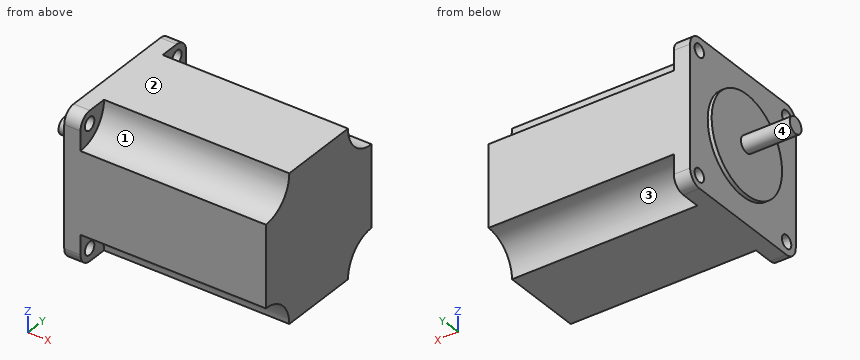
from build123d import *

# Parameters (mm, degrees)
SKETCH1_W           = 57.15
SKETCH1_H           = 57.15
SKETCH1_R           = 2.54
BOSS_EXTRUDE1_DEPTH = 6.35
FILLET1_R           = 5.08
SKETCH5_R           = 19.05
BOSS_EXTRUDE4_DEPTH = 1.524
SKETCH6_R           = 3.175
BOSS_EXTRUDE5_DEPTH = 19.05
BOSS_EXTRUDE6_DEPTH = 72.39


with BuildPart() as part:
    # Sketch1 → Boss-Extrude1 (new body)
    with BuildSketch(Plane(origin=(0, 0, 0), x_dir=(0, 0, -1), z_dir=(1, 0, 0))):
        Rectangle(SKETCH1_W, SKETCH1_H)
        with Locations((23.622, 23.622)):
            Circle(SKETCH1_R, mode=Mode.SUBTRACT)
        with Locations((-23.622, 23.622)):
            Circle(SKETCH1_R, mode=Mode.SUBTRACT)
        with Locations((-23.622, -23.622)):
            Circle(SKETCH1_R, mode=Mode.SUBTRACT)
        with Locations((23.622, -23.622)):
            Circle(SKETCH1_R, mode=Mode.SUBTRACT)
    extrude(amount=BOSS_EXTRUDE1_DEPTH)

    # Fillet1
    fillet1_edges = [part.edges().sort_by_distance(p)[0] for p in [
        (3.175, 28.575, 28.575),
        (3.175, 28.575, -28.575),
        (3.175, -28.575, -28.575),
        (3.175, -28.575, 28.575),
    ]]
    fillet(fillet1_edges, radius=FILLET1_R)

    # Sketch5 → Boss-Extrude4 (add)
    with BuildSketch(Plane.ZY):
        Circle(SKETCH5_R)
    extrude(amount=BOSS_EXTRUDE4_DEPTH)

    # Sketch6 → Boss-Extrude5 (add)
    with BuildSketch(Plane.ZY.offset(1.524)):
        Circle(SKETCH6_R)
    extrude(amount=BOSS_EXTRUDE5_DEPTH)

    # Sketch7 → Boss-Extrude6 (add)
    with BuildSketch(Plane(origin=(6.35, 0, 0), x_dir=(0, 0, -1), z_dir=(1, 0, 0))):
        with BuildLine():
            Line((-15.875, 28.575), (15.875, 28.575))
            ThreePointArc((15.875, 28.575), (19.594743879, 19.594743879), (28.575, 15.875))
            Line((28.575, 15.875), (28.575, -15.875))
            ThreePointArc((28.575, -15.875), (19.594743879, -19.594743879), (15.875, -28.575))
            Line((15.875, -28.575), (-15.875, -28.575))
            ThreePointArc((-15.875, -28.575), (-19.594743879, -19.594743879), (-28.575, -15.875))
            Line((-28.575, -15.875), (-28.575, 15.875))
            ThreePointArc((-28.575, 15.875), (-19.594743879, 19.594743879), (-15.875, 28.575))
        make_face()
    extrude(amount=BOSS_EXTRUDE6_DEPTH)


solid = part.part
Could you check a few things on this model? Use its own coordinates, in mm. Face numbers are marked on the shaded views. A direction names the side the tool comes from. Give positions to 0.01 mm unless a question says otherwise; leave off trailing zeros. Write each loop counter-clockwise with the first axis right and the second up, starting at its lowest first coordinate (ties: lowest second). Pieces come first, ordered by that corner, then holes. Notation, with made-up numbers: (21, 10.5) -> (51, 10.5) arc R6 cw to (51, 15.5) -> close; hole circle Ø11 at (59.25, -33.5). An arc over 180 degrees is marked (long way). Answer as a JSON object with one key per item and string values.
Q1. Will these pins go through, and if not, where does the flat tip stop? pin 1 Ø10 at (y, z) = (9, 2) entering from -X; pin 2 Ø1.5 at (y, z) = (9, 19.5) entering from -X; pin 3 Ø14 at (y, z) = (-23.5, 23.5) entering from +X; pin 4 Ø4 at (x, y) = (53.5, -21.5) entering from +Z.
Taken from the geometry:
{"pin 1": "stops at x = -1.52", "pin 2": "stops at x = 0", "pin 3": "stops at x = 78.74", "pin 4": "stops at z = 19.69"}
Q2. Which directions (+Z, -Z, +X, -X, +Y, -Y) give clear straight access to the entire face, cutting with the end or side of a thin tool? Please do the marked faces 1, 2, 3 and 4.
Taken from the geometry:
{"face 1": "+Z, +X, -Y", "face 2": "+Z, +X, -X, +Y, -Y", "face 3": "-Z, +X, +Y", "face 4": "-X"}
Q3. Suppose I cut it at C-C on z = 8.5. Write out the boundary of the cut face in (x, y) (3 decimals), then the cut area to 3 significant figures.
Taken from the geometry:
{"outline": "(-1.524, -17.049) -> (0, -17.049) -> (0, -28.575) -> (78.74, -28.575) -> (78.74, 28.575) -> (0, 28.575) -> (0, 17.049) -> (-1.524, 17.049) -> close", "area": "4,550 mm²"}
Q4. Suppose I cut it at A-A on y = 0. Write out the boundary of the cut face in (x, z) (3 decimals), then the cut area to 3 significant figures.
Taken from the geometry:
{"outline": "(-20.574, -3.175) -> (-1.524, -3.175) -> (-1.524, -19.05) -> (0, -19.05) -> (0, -28.575) -> (78.74, -28.575) -> (78.74, 28.575) -> (0, 28.575) -> (0, 19.05) -> (-1.524, 19.05) -> (-1.524, 3.175) -> (-20.574, 3.175) -> close", "area": "4,680 mm²"}
Q5. Please list where these lines run through material, in increasing order: L1, parallel to X at y = -13, z = -15; L2, parallel to X at y = -6, z = -0.5; L3, parallel to Y at x = 18, z = 25.5.
Taken from the geometry:
{"L1": "x = 0 to 78.74", "L2": "x = -1.52 to 78.74", "L3": "y = -16.25 to 16.25"}
Q6. Suppose I cut it at B-B on x = 26. Write out the boundary of the cut face in (y, z) (3 decimals).
Taken from the geometry:
{"outline": "(-28.575, -15.875) arc R12.7 cw to (-15.875, -28.575) -> (15.875, -28.575) arc R12.7 cw to (28.575, -15.875) -> (28.575, 15.875) arc R12.7 cw to (15.875, 28.575) -> (-15.875, 28.575) arc R12.7 cw to (-28.575, 15.875) -> close"}
